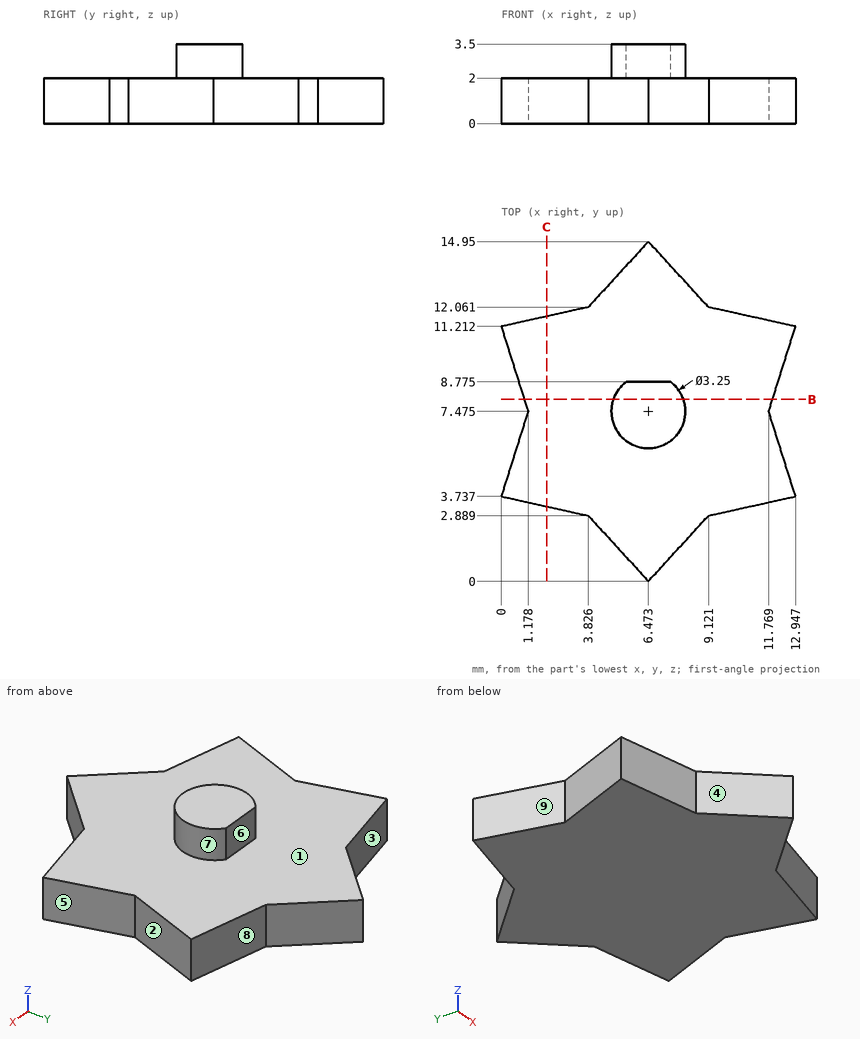
Geometry: see drawing. Coordinates: mm, zero at the bounding-box minimum. A direction names the side the tool comes from. Round coordinates to 2 decimals unless told otherwise and drop trailing zeros. Write each loop counter-clockwise with the first axis right and the second up, starting at its lowest first coordinate (ties: lowest second). Pieces come first, ordered by that corner, then holes.
Item 1: Pin query (flat end, axial travel): P1, Ø0.8, axis at x = 6.5, z = 3, coming from the +Y side (1 decimal). Return the tip coordinate at first contact, or that it passes through.
Item 2: Material intervals for L1, parallel to Z at x = 7.75, y = 9.5; L2, parallel to X at y = 8, z = 0.4 (1 decimal); L3, parallel to X at y = 8.5, z = 0.9 (1 decimal), sorted ascending.
Item 3: Set-up query: the marked faces 5, 6, 7, 8 and 9. Return all of +Z, -Z, +X, -X, +Y, -Y with unobstructed straight access to the full face (end or side cutting, diameter ignored); none if empty.
Item 4: Mould query, pull axis Y, two halves, no side actions, for the marked faces 1, 2, 3 and 4. Classes: +Y half, -Y half, draft (parallel to the pull), parting line (faces both ways), or undercut.
Item 5: Section query C-C (x = 2). Return loops of the section in (y, z) (1 decimal), plus the area to 3 significant figures.
Item 6: Section query B-B (y = 8). Return loops of the section in (x, z) (1 decimal).
Completed:
1. P1: stops at y = 8.8
2. L1: z = 0 to 2
2. L2: x = 1 to 11.9
2. L3: x = 0.9 to 12.1
3. face 5: +Z, -Z, +X
3. face 6: +Z, +X, -X, +Y
3. face 7: +Z
3. face 8: +Z, -Z, +X, +Y
3. face 9: +Z, -Z, -X
4. face 1: draft
4. face 2: undercut
4. face 3: +Y half
4. face 4: -Y half
5. outline: (3.3, 0) - (11.7, 0) - (11.7, 2) - (3.3, 2) - close
5. area: 16.7 mm2
6. outline: (1, 0) - (11.9, 0) - (11.9, 2) - (8, 2) - (8, 3.5) - (4.9, 3.5) - (4.9, 2) - (1, 2) - close
